from build123d import *

# Parameters (mm, degrees)
CROQUIS1_R                = 8.001
SALIENTE_EXTRUIR1_DEPTH   = 31.75
CROQUIS1_R_2              = 6.35
CROQUIS1_R_3              = 9.525
CROQUIS1_R_4              = 25.4
SALIENTE_EXTRUIR1_2_DEPTH = 31.75
SALIENTE_EXTRUIR2_DEPTH   = 82.55
CORTAR_EXTRUIR1_REACH     = 166.592
CROQUIS3_R                = 12.7
SALIENTE_EXTRUIR3_REACH   = 71.85


with BuildPart() as part:
    # Croquis1 → Saliente-Extruir1 (new body)
    with BuildSketch(Plane.XY):
        with BuildLine():
            Line((50.8, 170.942), (12.7, 170.942))
            Line((12.7, 170.942), (12.7, 154.94))
            Line((12.7, 154.94), (-12.7, 154.94))
            Line((-12.7, 154.94), (-12.7, 170.942))
            Line((-12.7, 170.942), (-50.8, 170.942))
            ThreePointArc((-50.8, 170.942), (-55.290128061, 169.082128061), (-57.15, 164.592))
            Line((-57.15, 164.592), (-57.15, 101.092))
            ThreePointArc((-57.15, 101.092), (-55.290128061, 105.582128061), (-50.8, 107.442))
            Line((-50.8, 107.442), (50.8, 107.442))
            ThreePointArc((50.8, 107.442), (55.290128061, 105.582128061), (57.15, 101.092))
            Line((57.15, 101.092), (57.15, 164.592))
            ThreePointArc((57.15, 164.592), (55.290128061, 169.082128061), (50.8, 170.942))
        make_face()
        with Locations((-28.448, 136.652)):
            Circle(CROQUIS1_R, mode=Mode.SUBTRACT)
        with Locations((28.448, 135.89)):
            Circle(CROQUIS1_R, mode=Mode.SUBTRACT)
    extrude(amount=SALIENTE_EXTRUIR1_DEPTH)



with BuildPart() as body_2:
    # Croquis1 → Saliente-Extruir1 2 (new body)
    with BuildSketch(Plane.XY):
        with BuildLine():
            Line((57.15, 0), (57.15, 75.692))
            ThreePointArc((57.15, 75.692), (55.290128061, 71.201871939), (50.8, 69.342))
            Line((50.8, 69.342), (-50.8, 69.342))
            ThreePointArc((-50.8, 69.342), (-55.290128061, 71.201871939), (-57.15, 75.692))
            Line((-57.15, 75.692), (-57.15, 0))
            ThreePointArc((-57.15, 0), (0, -57.15), (57.15, 0))
        make_face()
        with Locations((-28.702, 41.402)):
            Circle(CROQUIS1_R_2, mode=Mode.SUBTRACT)
        with Locations((0, -41.402)):
            Circle(CROQUIS1_R_3, mode=Mode.SUBTRACT)
        Circle(CROQUIS1_R_4, mode=Mode.SUBTRACT)
    extrude(amount=SALIENTE_EXTRUIR1_2_DEPTH)


with BuildPart() as part_1:
    add(part.part)

    add(body_2.part)  # Saliente-Extruir2 merges body 2
    # Croquis1_3 → Saliente-Extruir2 (add)
    with BuildSketch(Plane.XY):
        with BuildLine():
            Line((57.15, 75.692), (57.15, 101.092))
            ThreePointArc((57.15, 101.092), (55.290128061, 105.582128061), (50.8, 107.442))
            Line((50.8, 107.442), (-50.8, 107.442))
            ThreePointArc((-50.8, 107.442), (-55.290128061, 105.582128061), (-57.15, 101.092))
            Line((-57.15, 101.092), (-57.15, 75.692))
            ThreePointArc((-57.15, 75.692), (-55.290128061, 71.201871939), (-50.8, 69.342))
            Line((-50.8, 69.342), (50.8, 69.342))
            ThreePointArc((50.8, 69.342), (55.290128061, 71.201871939), (57.15, 75.692))
        make_face()
    extrude(amount=SALIENTE_EXTRUIR2_DEPTH)

    # Croquis3 → Cortar-Extruir1 (cut, up to next)
    with BuildSketch(Plane(origin=(0, 107.442, 0), x_dir=(1, 0, 0), z_dir=(0, 1, 0)), mode=Mode.PRIVATE) as cortar_extruir1_sk1:
        with Locations((0, -57.15)):
            Circle(CROQUIS3_R)
    cortar_extruir1_tool1 = extrude(cortar_extruir1_sk1.sketch, amount=-CORTAR_EXTRUIR1_REACH, mode=Mode.PRIVATE) & part_1.part
    add(cortar_extruir1_tool1.solids().sort_by_distance((0, 107.442, 57.15))[0], mode=Mode.SUBTRACT)

    # Croquis4 → Saliente-Extruir3 (add, up to next)
    with BuildSketch(Plane.ZY.offset(-12.7), mode=Mode.PRIVATE) as saliente_extruir3_sk1:
        Polygon((31.75, 154.94), (0, 170.942), (0, 154.94), align=None)
    saliente_extruir3_tool1 = extrude(saliente_extruir3_sk1.sketch, amount=SALIENTE_EXTRUIR3_REACH, mode=Mode.PRIVATE) - part_1.part
    add(saliente_extruir3_tool1.solids().sort_by_distance((12.7, 160.274, 10.583333))[0])


solid = part_1.part
Could you check a few things on this model? Use its own coordinates, in mm. A direction names the side the tool comes from. Give positions to 0.01 mm unless a question says otherwise; leave off trailing zeros. Order: outer loops, then holes, each group sorted by start corner. A loop starts at its lowest first (then second) coordinate and runs counter-clockwise, first axis right, second up. Notation, with made-up numbers: (36, -39) - (74, -39) arc R25 cw to (74, -11) - close; hole circle Ø6 at (18, -40). An arc over 180 degrees is marked (long way). Return JSON: item names as keys, results as strings. Group by question number.
Q1. Suppose I cut it at D-D, the plane y = 116.5. Please give me the cut outline in (x, z).
Q2. Suppose I cut it at A-A, the plane x = 0. Please give me the cut outline in (y, z), and give its area (3 significant figures).
Q3. Which directions (+Z, -Z, +X, -X, +Y, -Y) give clear straight access to the entire face, cutting with the end or side of a thin tool? Please do faces 5 (the face through (-55.24, 105.63, 56.79)), 6 (the face through (-1, 89, 82.55)), 7 (the face through (-12.7, 166, 23)), 8 (the face through (-12, 69.342, 51)).
Q4. Suppose I cut it at B-B, the plane z = 57.15. Please give me the cut outline in (x, y), and give its area (3 significant figures).
Q5. Suppose I cut it at C-C, the plane y = 73. Please give me the cut outline in (x, z).
Q6. Will these pins go through, and if not, where does the flat tip stop? pin 1 Ø20.5 at (x, y) = (-28.702, 41.402) entering from +Z; pin 2 Ø15 at (x, z) = (-14.5, 57) entering from +Y; pin 3 Ø10 at (x, z) = (-8.5, 73) entering from -Y.
Q7. Please list where these lines run through material, in increasing order: line 1 along Z through (x, y) = (0, 88); line 2 along Y through (x, z) = (0, 10); line 3 along Y through (x, z) = (0, 17.5). Write a range as [from, to].
Q8. Thinking about a two-plate mould opening in Y: for faces 1 (the face through (26.71, 128.08, 15.65)), 2 (the face through (55.34, 169.03, 15.65)), 3 (the face through (-5.506, -24.796, 15.653)), 4 (the face through (12.7, 167, 23)), which applies, pulls with the +Y half, pulls with the -Y half, needs draft (parallel to the pull), parting line crosses it, or undercut?
Resolved:
{
 "1": {"outline": "(-57.15, 0) - (57.15, 0) - (57.15, 31.75) - (-57.15, 31.75) - close"},
 "2": {"outline": "(-57.15, 0) - (-50.93, 0) - (-50.93, 31.75) - (-57.15, 31.75) - close; (-31.88, 0) - (-25.4, 0) - (-25.4, 31.75) - (-31.88, 31.75) - close; (25.4, 0) - (170.94, 0) - (154.94, 31.75) - (107.44, 31.75) - (107.44, 44.45) - (69.34, 44.45) - (69.34, 31.75) - (25.4, 31.75) - close; (69.34, 69.85) - (107.44, 69.85) - (107.44, 82.55) - (69.34, 82.55) - close", "area": "5,740 mm2"},
 "3": {"face 5": "+Z, -X, +Y", "face 6": "+Z, +X, -X, +Y, -Y", "face 7": "+Z, +Y", "face 8": "+Z, +X, -X, -Y"},
 "4": {"outline": "(-57.15, 75.69) arc R6.35 ccw to (-50.8, 69.34) - (-12.7, 69.34) - (-12.7, 107.44) - (-50.8, 107.44) arc R6.35 ccw to (-57.15, 101.09) - close; (12.7, 69.34) - (50.8, 69.34) arc R6.35 ccw to (57.15, 75.69) - (57.15, 101.09) arc R6.35 ccw to (50.8, 107.44) - (12.7, 107.44) - close", "area": "3,350 mm2"},
 "5": {"outline": "(-57.15, 0) - (57.15, 0) - (57.15, 31.75) - (56.55, 31.75) - (56.55, 82.55) - (-56.55, 82.55) - (-56.55, 31.75) - (-57.15, 31.75) - close; hole circle Ø25.4 at (0, 57.15)"},
 "6": {"pin 1": "stops at z = 31.75", "pin 2": "stops at y = 107.44", "pin 3": "stops at y = 69.34"},
 "7": {"line 1": "z = [0, 44.45], [69.85, 82.55]", "line 2": "y = [-57.15, -50.93], [-31.88, -25.4], [25.4, 165.9]", "line 3": "y = [-57.15, -50.93], [-31.88, -25.4], [25.4, 162.12]"},
 "8": {"face 1": "undercut", "face 2": "pulls with the +Y half", "face 3": "undercut", "face 4": "needs draft"}
}
